Autodesk Inventor part; units mm, degrees
ref_plane "YZ Plane" through (0, 0, 0) normal (1, 0, 0) x (0, 1, 0)
ref_plane "XZ Plane" through (0, 0, 0) normal (0, 1, 0) x (-1, 0, 0)
ref_plane "XY Plane" through (0, 0, 0) normal (0, 0, 1) x (1, 0, 0)
sketch "Sketch1" plane through (0, 0, 0) normal (0, 0, 1) x (1, 0, 0)
  line L0 (13.335, -13.335) -> (-13.335, -13.335)
  line L1 (-13.335, -13.335) -> (-13.335, 13.335)
  line L2 (-13.335, 13.335) -> (13.335, 13.335)
  line L3 (13.335, 13.335) -> (13.335, -13.335)
  line L4 (13.335, -13.335) -> (-13.335, 13.335) construction
  line L5 (-13.335, -13.335) -> (13.335, 13.335) construction
  line L6 (15.24, -15.24) -> (-15.24, -15.24)
  line L7 (-15.24, -15.24) -> (-15.24, 15.24)
  line L8 (-15.24, 15.24) -> (15.24, 15.24)
  line L9 (15.24, 15.24) -> (15.24, -15.24)
  line L10 (15.24, -15.24) -> (-15.24, 15.24) construction
  line L11 (-15.24, -15.24) -> (15.24, 15.24) construction
  point P0 (0, 0)
  dimension "d0" = 26.67
  dimension "d1" = 26.67
  dimension "d2" = 30.48
  dimension "d3" = 30.48
extrude "Extrusion1" add sketch "Sketch1" along normal blind 31.75
extrude "Extrusion2" add sketch "Sketch1" along normal blind 6.35 contours L0 L1 L2 L3
sketch "Sketch2" plane through (-15.24, 15.24, 0) normal (0, 1, 0) x (1, 0, 0)
  line L0 (1.905, -6.35) -> (28.575, -6.35)
  line L1 (30.48, 0) -> (0, 0)
  line L2 (0, 0) -> (0, -31.75)
  line L3 (30.48, -31.75) -> (0, -31.75)
  line L4 (30.48, 0) -> (30.48, -31.75)
  line L5 (15.24, 0) -> (15.24, -31.75) construction
  line L6 (28.575, -31.75) -> (1.905, -31.75) construction
  circle A0 centre (15.24, -19.05) radius 2.25
  circle A1 centre (15.24, -25.4) radius 2.25
  dimension "d8" = 4.5
  dimension "d9" = 12.7
  dimension "d10" = 4.5
  dimension "d11" = 6.35
extrude "Extrusion3" cut sketch "Sketch2" against normal up to surface (28.575 mm away) contours A0 | A1
sketch "Sketch3" plane through (-15.24, -15.24, 0) normal (0, -1, 0) x (1, 0, 0)
  circle A0 centre (15.24, 19.05) radius 2.25
  line L0 (0, 0) -> (30.48, 0)
  line L1 (30.48, 0) -> (30.48, 31.75)
  line L2 (0, 31.75) -> (30.48, 31.75)
  line L3 (0, 0) -> (0, 31.75)
  circle A1 centre (15.24, 25.4) radius 2.25
  circle A2 centre (15.24, 25.4) radius 1.5
  circle A3 centre (15.24, 19.05) radius 1.5
  point P0 (15.24, 0)
  dimension "d14" = 3
  dimension "d15" = 3
extrude "Extrusion4" cut sketch "Sketch3" against normal up to surface (28.575 mm away) contours A2 | A3
properties part number "CS_Climb_Inner_Tube_End_Cap"
Could you check a few things on this model? Use its own coordinates, in mm. A direction names the side the tool comes from. Coordinates: 2 decimals unless noted, no trailing zeros. Loops run counter-clockwise (first coordinate to the right, second up) from the corner with the lowest first, then second, coordinate; pieces in that order, holes last. Notation, with made-up numbers: M 9,-14.5 L 51,-14.5 A38 cw 51,23.5 Z; hole C 64.5,45.25 d4. An arc over 180 degrees is marked long. Put each result on its own line as item: value. Start each with the question number.
(1) Suppose I cut it at A-A on z = 25.4. Please give me the cut outline in (x, y) (3 decimals).
(2) Thinking about a two-plate mould opening in X: for faces 1 (the face through (0, 15.24, 16)), 2 (the face through (-15.24, 0, 16)), 3 (the face through (-0.488, 14.301, 21.246)), 4 (the face through (-13.335, 0, 19)), which applies, pulls with the +X half, pulls with the -X half, needs draft (parallel to the pull), parting line crosses it, or undercut?
(3) For faces 5 (the face through (0, -13.335, 16)), 6 (the face through (0, 0, 0)), 7 (the face through (-0.29, 14.3, 23.17)), which set-ups out of +Z, -Z, +X, -X, +Y, -Y let a thin tool reach every point of the face, with its end or its side?
(4) Will these pins go through, and if not, where does the flat tip stop? P1, Ø3.5, axis at x = 0, z = 25.4, coming from the +Y side (3 decimals); P2, Ø12, axis at x = -11, y = 2.5, coming from the +Z side; P3, Ø2, axis at x = 9, y = 11, coming from the +Z side.
(5) Suppose I cut it at C-C on y = 10. Please give me the cut outline in (x, z) (3 decimals), then the cut area to 3 significant figures.
(6) Suppose I cut it at B-B on x = 0. Please give me the cut outline in (y, z) (3 decimals).
(7) I need wall thicknesses on line 1 (Z direction, x = 0, y = -14.8); line 2 (Y direction, x = -11, z = 10) (3 decimals). Which ranges of each line are inside material? Lowest first, please. Write a range as from..to.
(8) Suppose I cut it at D-D on z = 16. Please give me the cut outline in (x, y) (3 decimals).
Solutions:
1. outline: M -15.24,-15.24 L -1.5,-15.24 L -1.5,-13.335 L -13.335,-13.335 L -13.335,13.335 L -2.25,13.335 L -2.25,15.24 L -15.24,15.24 Z; M 1.5,-15.24 L 15.24,-15.24 L 15.24,15.24 L 2.25,15.24 L 2.25,13.335 L 13.335,13.335 L 13.335,-13.335 L 1.5,-13.335 Z
2. face 1: needs draft
2. face 2: pulls with the -X half
2. face 3: undercut
2. face 4: undercut
3. face 5: +Z
3. face 6: -Z, +X, -X, +Y, -Y
3. face 7: +Y
4. P1: stops at y = -13.335
4. P2: stops at z = 31.75
4. P3: stops at z = 6.35
5. outline: M -15.24,0 L 15.24,0 L 15.24,31.75 L 13.335,31.75 L 13.335,6.35 L -13.335,6.35 L -13.335,31.75 L -15.24,31.75 Z
5. area: 290 mm2
6. outline: M -15.24,0 L 15.24,0 L 15.24,16.8 L 13.335,16.8 L 13.335,6.35 L -13.335,6.35 L -13.335,17.55 L -15.24,17.55 Z; M -15.24,20.55 L -13.335,20.55 L -13.335,23.9 L -15.24,23.9 Z; M -15.24,26.9 L -13.335,26.9 L -13.335,31.75 L -15.24,31.75 Z; M 13.335,21.3 L 15.24,21.3 L 15.24,23.15 L 13.335,23.15 Z; M 13.335,27.65 L 15.24,27.65 L 15.24,31.75 L 13.335,31.75 Z
7. line 1: z = 0..17.55, 20.55..23.9, 26.9..31.75
7. line 2: y = -15.24..-13.335, 13.335..15.24
8. outline: M -15.24,-15.24 L 15.24,-15.24 L 15.24,15.24 L -15.24,15.24 Z; hole M -13.335,-13.335 L 13.335,-13.335 L 13.335,13.335 L -13.335,13.335 Z
